Read the model definition and answer for the solid it produces. Units are mm, in the model's axes. A direction names the side the tool comes from. Round coordinates to 2 decimals unless told otherwise and drop trailing zeros. Order: outer loops, then holes, each group sorted by start corner. A loop starts at its lowest first (then second) coordinate and runs counter-clockwise, first axis right, second up. Notation, with made-up numbers: M -33.75,-26 L -13.75,-26 A11 cw -13.75,-15 Z; hole C 17,-36 d1. An arc over 180 degrees is marked long. Answer as CSV lines item,"result".
```python
from build123d import *

# Parameters (mm, degrees)
SKETCH1_W          = 171
SKETCH1_H          = 113
EXTRUDE1_DEPTH     = 22
EXTRUDE2_START     = -3
EXTRUDE2_OUTLINE_W = 154
EXTRUDE2_OUTLINE_H = 85.5
EXTRUDE2_DEPTH     = 3
SKETCH3_R          = 2.75
EXTRUDE3_DEPTH     = 10


# Read off the part's stored shape, not the designer's step: Extrude2
with BuildPart() as part:
    # Sketch1 → Extrude1 (new body)
    with BuildSketch(Plane.XY):
        Rectangle(SKETCH1_W, SKETCH1_H)
    extrude(amount=EXTRUDE1_DEPTH)

    # Extrude2 outline → Extrude2 (cut)
    with BuildSketch(Plane.XY.offset(22).offset(EXTRUDE2_START)):
        with Locations((0, 1.25)):
            Rectangle(EXTRUDE2_OUTLINE_W, EXTRUDE2_OUTLINE_H)
    extrude(amount=EXTRUDE2_DEPTH, mode=Mode.SUBTRACT)

    # Sketch3 → Extrude3 (cut)
    with BuildSketch(Plane.XZ.offset(56.5)):
        with Locations((0, 8.5)):
            Circle(SKETCH3_R)
    extrude(amount=-EXTRUDE3_DEPTH, mode=Mode.SUBTRACT)


solid = part.part
```
Item 1: A cutting plane is placed at B-B, the plane x = 0. Determine the outline of the cut face in (y, z), and give its area (3 significant figures).
Ans:
outline,"M -56.5,0 L 56.5,0 L 56.5,22 L 44,22 L 44,19 L -41.5,19 L -41.5,22 L -56.5,22 L -56.5,11.25 L -46.5,11.25 L -46.5,5.75 L -56.5,5.75 Z"
area,"2,170 mm2"
Item 2: A cutting plane is placed at A-A, the plane y = 15. Determine the outline of the cut face in (x, z).
Ans:
outline,"M -85.5,0 L 85.5,0 L 85.5,22 L 77,22 L 77,19 L -77,19 L -77,22 L -85.5,22 Z"
Item 3: Find the intervals of material crossed by probe 1 along Z at (x, y) = (0, -53.5); probe 2 along Z at (x, y) = (29, 34), in increasing order. Write a range as [from, to].
Ans:
probe 1,"[0, 5.75], [11.25, 22]"
probe 2,"[0, 19]"
Item 4: Determine the mould class of faces 1 (the face through (-1, 56.5, 11)), 2 (the face through (-1, 2, 19)), 3 (the face through (-85.5, -1, 11)) for opening direction X: +X half, -X half, draft (parallel to the pull), parting line (faces both ways), or undercut.
Ans:
face 1,"draft"
face 2,"undercut"
face 3,"-X half"
Item 5: Flat-ended cylindrical pins translate along their axes: pin 1 (2 mm diameter, centred on x = 66.5, y = 1, fed in from +Z); pin 2 (1.6 mm diameter, centred on x = 0, z = 8, fed in from -Y). Find the tip coordinate at first contact, or state that the pin passes through.
Ans:
pin 1,"z = 19"
pin 2,"y = -46.5"
Item 6: A tool of negligible diameter and unlimited length cuts with its end or side. For faces 4 (the face through (-2.027, -51.57, 10.359)), 5 (the face through (85.5, -1, 11)), from which of +Z, -Z, +X, -X, +Y, -Y can it reach the whole face along a straight path? Write none if from no direction.
Ans:
face 4,"-Y"
face 5,"+Z, -Z, +X, +Y, -Y"
Item 7: A cutting plane is placed at C-C, the plane x = 42. Determine the outline of the cut face in (y, z), and give its area (3 significant figures).
Ans:
outline,"M -56.5,0 L 56.5,0 L 56.5,22 L 44,22 L 44,19 L -41.5,19 L -41.5,22 L -56.5,22 Z"
area,"2,230 mm2"
